```python
from build123d import *

# Parameters (mm, degrees)
F1_DEPTH  = 12
F3_DEPTH  = 40
F4_R      = 20
F4_R_2    = 10.076215
F5_DEPTH  = 28
F5_FACE_R = 10.076215
F6_DEPTH  = 25


with BuildPart() as f1:
    # F0 (on Front) → F1 (new body)
    with BuildSketch(Plane.XZ):
        with BuildLine():
            Line((-44, 40), (-44, 0))
            Line((-44, 0), (44, 0))
            Line((44, 0), (44, 40))
            ThreePointArc((44, 40), (0, 84), (-44, 40))
        make_face()
    extrude(amount=F1_DEPTH)

    # F2 (on Front) → F3 (join)
    with BuildSketch(Plane.XZ):
        Polygon((44, 0), (-44, 0), (-44, -29.557653), (-22, -29.557653), (-22, -14.557653), (22, -14.557653), (22, -29.557653), (44, -29.557653), align=None)
    extrude(amount=F3_DEPTH)

    # F4 (on Front) → F5 (join)
    with BuildSketch(Plane.XZ):
        with Locations((0, 40)):
            Circle(F4_R)
        with Locations((0, 40)):
            Circle(F4_R_2, mode=Mode.SUBTRACT)
    extrude(amount=F5_DEPTH)

    # F5_face (on face) → F6 (cut)
    with BuildSketch(Plane(origin=(0, -12, 40), x_dir=(1, 0, 0), z_dir=(0, -1, 0))):
        Circle(F5_FACE_R)
    extrude(amount=-F6_DEPTH, mode=Mode.SUBTRACT)


solid = f1.part
```
Read the model definition and answer for the solid it produces. Units are mm, in the model's axes. A direction names the side the tool comes from. Round coordinates to 2 decimals unless told otherwise and drop trailing zeros. Write each loop counter-clockwise with the first axis right and the second up, starting at its lowest first coordinate (ties: lowest second). Pieces come first, ordered by that corner, then holes. Notation, with made-up numbers: (-22.5, 59) -> (3.5, 59) arc R29 cw to (3.5, 86) -> close; hole circle Ø2 at (45.25, -14). An arc over 180 degrees is marked (long way). Answer in a Markdown table with one row per item. Add a question column.
1) Find section A-A, the plane x = 0. Determine the outline of the cut face in (y, z).
2) Find section C-C, the plane z = 47. Determine the outline of the cut face in (x, y) (3 decimals), and give its area (3 significant figures).
3) Find section B-B, the plane y = -31.5. Determine the outline of the cut face in (x, z).
4) Consider line 1 (Z direction, x = 0, y = -22); line 2 (Z direction, x = 2.5, y = -25); line 3 (Z direction, x = 0, y = -8). Determine where each line is inside the solid, lowest interval first.
5) Determine the mould class of faces 1 (the face through (-2.6, -19.89, 59.83)), 2 (the face through (44, -15, -3)), 3 (the face through (1, -26, 0)), 4 (the face through (0, -20, -14.558)) for opening direction Z: pulls with the +Z half, pulls with the -Z half, needs draft (parallel to the pull), parting line crosses it, or undercut.
6) Which of the six approach directions +Z, -Z, +X, -X, +Y, -Y give full straight-line access (tool end or side, diameter ignored) to faces 5 (the face through (22, -20, -22)), 6 (the face through (-5, -28, 49)), 7 (the face through (19, -12, 33))?
7) Find section D-D, the plane y = -5. Determine the outline of the cut face in (x, z).
8) Given P1, Ø6, axis at x = 8, z = 23.5, coming from the -Y side; P2, Ø4, axis at x = -15, y = -12, coming from the +Z side; P3, Ø8.5, axis at x = 15, y = -27.5, coming from the +Z side, each flat-ended and moving along its own axis, determine where each tip first touches the part or whether it passes through.
Findings below:
| question | item | result |
|---|---|---|
| 1 | outline | (-40, -14.56) -> (0, -14.56) -> (0, 29.92) -> (-28, 29.92) -> (-28, 20) -> (-12, 20) -> (-12, 0) -> (-40, 0) -> close; (-28, 50.08) -> (0, 50.08) -> (0, 84) -> (-12, 84) -> (-12, 60) -> (-28, 60) -> close |
| 2 | outline | (-43.44, -12) -> (-18.735, -12) -> (-18.735, -28) -> (-7.248, -28) -> (-7.248, 0) -> (-43.44, 0) -> close; (7.248, -28) -> (18.735, -28) -> (18.735, -12) -> (43.44, -12) -> (43.44, 0) -> (7.248, 0) -> close |
| 2 | area | 1,240 mm² |
| 3 | outline | (-44, -29.56) -> (-22, -29.56) -> (-22, -14.56) -> (22, -14.56) -> (22, -29.56) -> (44, -29.56) -> (44, 0) -> (-44, 0) -> close |
| 4 | line 1 | -14.56 to 0, 20 to 29.92, 50.08 to 60 |
| 4 | line 2 | -14.56 to 0, 20.16 to 30.24, 49.76 to 59.84 |
| 4 | line 3 | -14.56 to 29.92, 50.08 to 84 |
| 5 | face 1 | undercut |
| 5 | face 2 | needs draft |
| 5 | face 3 | undercut |
| 5 | face 4 | pulls with the -Z half |
| 6 | face 5 | -Z, +Y, -Y |
| 6 | face 6 | +Z, +X, -X, -Y |
| 6 | face 7 | -Y |
| 7 | outline | (-44, -29.56) -> (-22, -29.56) -> (-22, -14.56) -> (22, -14.56) -> (22, -29.56) -> (44, -29.56) -> (44, 40) arc R44 ccw to (-44, 40) -> close; hole circle Ø20.15 at (0, 40) |
| 8 | P1 | y = -28 |
| 8 | P2 | z = 82.04 |
| 8 | P3 | z = 56.87 |
